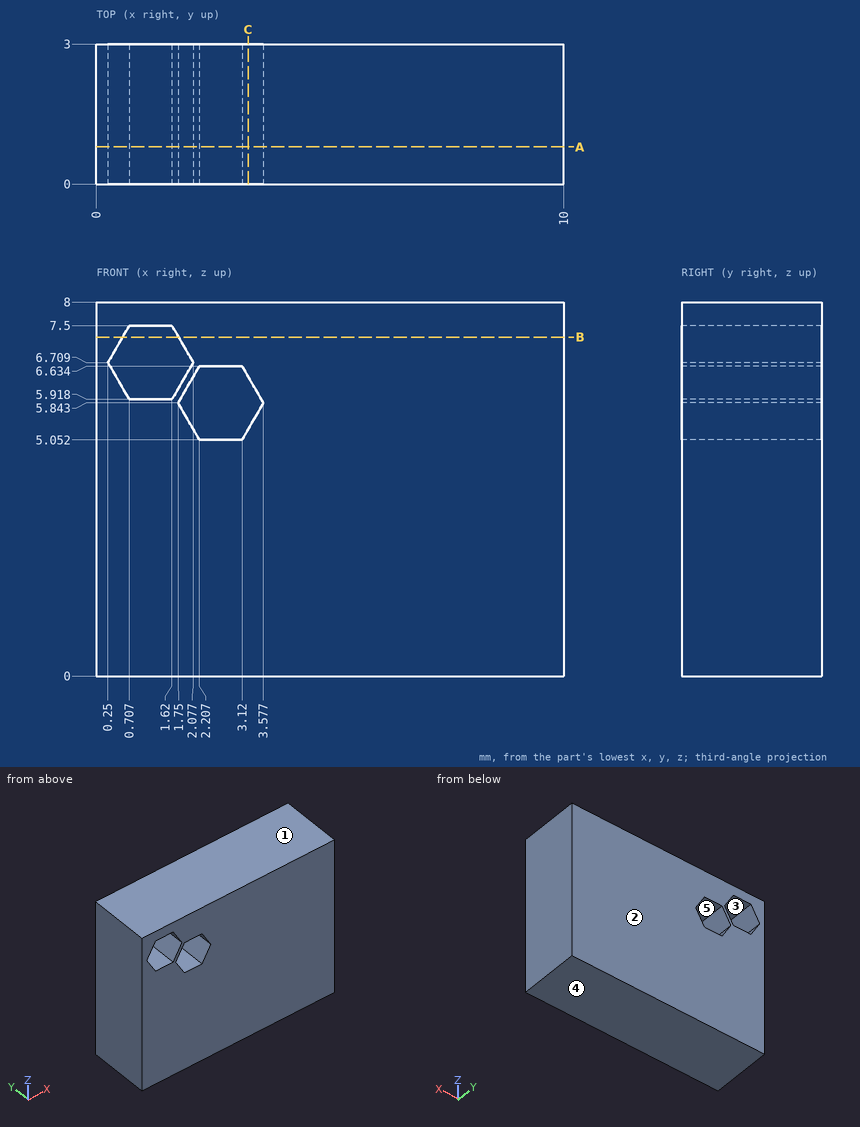
Answer from the drawing. Dimensions are ordinates in mm from the lowest x, y and z of the part. A direction names the side the tool comes from. Coordinates: 2 decimals unless noted, no trailing zeros. Order: outer loops, then holes, each group sorted by start corner. A loop starts at its lowest first (then second) coordinate and runs counter-clockwise, first axis right, second up. Notation, with made-up numbers: (55.5, 28.5) - (92.5, 28.5) arc R11 cw to (92.5, 47.5) - close; hole circle Ø11 at (-29, 73). An arc over 180 degrees is marked (long way). Put each result on its own line as item: value. Start each with the question number.
1) Find the intervals of material crossed by line 1 (Z direction, x = 2.5, y = 0.2); line 2 (X direction, y = 2.7, z = 6.25) (1 decimal); line 3 (Z direction, x = 2, y = 0.75) (1 decimal), in increasing order. Write a range as from..to.
2) Find section B-B (z = 7.25). Give the vertices of the cut face in (x, y) (1 decimal).
3) Find section C-C (x = 3.25). Give the vertices of the cut face in (y, z), plus the area to 3 significant figures.
4) Find section A-A (y = 0.8). Give the vertices of the cut face in (x, z).
5) For a pull along Z with two mould halves and no side action, classify the marked faces 1, 2 and 3 as released by +Z, released by -Z, zero draft, split by the parting line, or undercut.
6) For the marked faces 4 and 5, determine the directions among +Z, -Z, +X, -X, +Y, -Y from which every point of the face is accessible in a straight line to the end or side of a thin tool.
Results list:
1. line 1: z = 0..5.05, 6.63..8
1. line 2: x = 0..0.5, 1.8..2, 3.3..10
1. line 3: z = 0..5.4, 6.3..6.6, 6.8..8
2. outline: (0, 0) - (0.6, 0) - (0.6, 3) - (0, 3) - close; (1.8, 0) - (10, 0) - (10, 3) - (1.8, 3) - close
3. outline: (0, 0) - (3, 0) - (3, 5.28) - (0, 5.28) - close; (0, 6.41) - (3, 6.41) - (3, 8) - (0, 8) - close
3. area: 20.6 mm^2
4. outline: (0, 0) - (10, 0) - (10, 8) - (0, 8) - close; hole (0.25, 6.71) - (0.71, 5.92) - (1.62, 5.92) - (2.08, 6.71) - (1.62, 7.5) - (0.71, 7.5) - close; hole (1.75, 5.84) - (2.21, 5.05) - (3.12, 5.05) - (3.58, 5.84) - (3.12, 6.63) - (2.21, 6.63) - close
5. face 1: released by +Z
5. face 2: zero draft
5. face 3: undercut
6. face 4: -Z, +X, -X, +Y, -Y
6. face 5: +Y, -Y
